```python
from build123d import *

# Parameters (mm, degrees)
SKETCH_1_W             = 68.22
SKETCH_1_H             = 22
SM_BASE_FLANGE_1_DEPTH = 1
FILLET_1_R             = 1
OTHER_START            = -15.667913645
OTHER_1_DEPTH          = 22
OTHER_1_2_DEPTH        = 22
OTHER_START_2          = 27.250753262
OTHER_1_3_DEPTH        = 1.749246738
SKETCH_7_R             = 2
CUT_EXTRUDE_1_DEPTH    = 40
SKETCH_7_6_R           = 1.7
CUT_EXTRUDE_4_DEPTH    = 20


with BuildPart() as part:
    # 基体-法兰1: sheet metal written as solids
    # Sketch 1 → 基体-法兰1 (new body)
    with BuildSketch(Plane(origin=(0, 0, 0), x_dir=(1, 0, 0), z_dir=(0, 1, 0))):
        with Locations((-53.201792275, 4.667913645)):
            Rectangle(SKETCH_1_W, SKETCH_1_H)
    extrude(amount=-SM_BASE_FLANGE_1_DEPTH)

    # 圆角1
    fillet_1_edges = [part.edges().sort_by_distance(p)[0] for p in [
        (-87.311792275, -0.5, -15.667913645),
        (-19.091792275, -0.5, -15.667913645),
        (-19.091792275, -0.5, 6.332086355),
        (-87.311792275, -0.5, 6.332086355),
    ]]
    fillet(fillet_1_edges, radius=FILLET_1_R)

    # Other 1: read off the stored shape, not the designer's step
    # Other 1 outline → Other 1 (cut)
    with BuildSketch(Plane.XY.offset(OTHER_START)):
        with BuildLine():
            Line((-19.091792275, 0), (-53.739151185, 0))
            ThreePointArc((-53.739151185, 0), (-54.379966111, -0.728828115), (-55.311792275, -1))
            Line((-55.311792275, -1), (-19.091792275, -1))
            Line((-19.091792275, -1), (-19.091792275, 0))
        make_face()
    extrude(amount=OTHER_1_DEPTH, mode=Mode.SUBTRACT)

    # Other 1 2 outline → Other 1 2 (add)
    with BuildSketch(Plane.XY.offset(OTHER_START)):
        with BuildLine():
            ThreePointArc((-53.739151185, 0), (-53.616677518, 0.359286442), (-53.575192275, 0.7366))
            Line((-53.575192275, 0.7366), (-53.575192275, 26.514153262))
            ThreePointArc((-53.575192275, 26.514153262), (-54.083830639, 27.742114898), (-55.311792275, 28.250753262))
            Line((-55.311792275, 28.250753262), (-61.869345538, 28.250753262))
            Line((-61.869345538, 28.250753262), (-61.869345538, 27.250753262))
            Line((-61.869345538, 27.250753262), (-55.311792275, 27.250753262))
            ThreePointArc((-55.311792275, 27.250753262), (-54.79093742, 27.035008117), (-54.575192275, 26.514153262))
            Line((-54.575192275, 26.514153262), (-54.575192275, 0.7366))
            ThreePointArc((-54.575192275, 0.7366), (-54.79093742, 0.215745145), (-55.311792275, 0))
            Line((-55.311792275, 0), (-53.739151185, 0))
        make_face()
    extrude(amount=OTHER_1_2_DEPTH)

    # Other 1 3 outline → Other 1 3 (cut)
    with BuildSketch(Plane(origin=(0, 0, 0), x_dir=(1, 0, 0), z_dir=(0, 1, 0)).offset(OTHER_START_2)):
        with BuildLine():
            Line((-61.869345538, -6.332086355), (-60.869345538, -6.332086355))
            ThreePointArc((-60.869345538, -6.332086355), (-61.576452319, -6.039193136), (-61.869345538, -5.332086355))
            Line((-61.869345538, -5.332086355), (-61.869345538, -6.332086355))
        make_face()
        with BuildLine():
            Line((-61.869345538, 15.667913645), (-61.869345538, 14.667913645))
            ThreePointArc((-61.869345538, 14.667913645), (-61.576452319, 15.375020426), (-60.869345538, 15.667913645))
            Line((-60.869345538, 15.667913645), (-61.869345538, 15.667913645))
        make_face()
    extrude(amount=OTHER_1_3_DEPTH, mode=Mode.SUBTRACT)

    # 草图7 → 切除-拉伸1 (cut)
    with BuildSketch(Plane(origin=(0, 28.250753262, 0), x_dir=(1, 0, 0), z_dir=(0, 1, 0))):
        with Locations(Location((-80.654608631, -2.961737693, 0), (0, 0, 90))):
            Circle(SKETCH_7_R)
    extrude(amount=-CUT_EXTRUDE_1_DEPTH, mode=Mode.SUBTRACT)

    # 草图7<6> → 切除-拉伸4 (cut)
    with BuildSketch(Plane(origin=(0, 28.250753262, 0), x_dir=(1, 0, 0), z_dir=(0, 1, 0))):
        with Locations(Location((-58.548227621, 10.901663137, 0), (0, 0, 180))):
            Circle(SKETCH_7_6_R)
        with Locations(Location((-58.548227621, 0.801663137, 0), (0, 0, 180))):
            Circle(SKETCH_7_6_R)
    extrude(amount=-CUT_EXTRUDE_4_DEPTH, mode=Mode.SUBTRACT)


solid = part.part
```
Geometry check sheet. Reference: the model listing, model coordinates, mm. A direction names the side the tool comes from. Coordinates: 2 decimals unless noted, no trailing zeros. Order: outer loops, then holes, each group sorted by start corner. A loop starts at its lowest first (then second) coordinate and runs counter-clockwise, first axis right, second up.
Item 1: Tool access check on faces 1 (the cylindrical face through (-61.58, 27.74, -15.37)), 2 (the cylindrical face through (-61.569, 27.744, 6.047)), 3 (the cylindrical face through (-57.3, 27.76, -9.75)), 4 (the flat face through (-61.869, 28, -5)), 5 (the flat face through (-54.575, 14, -5)). Record the directions out of +Z, -Z, +X, -X, +Y, -Y that give a thin tool (end or side, any length) a straight path to the whole face; none if there is none.
Item 2: Depth check by flat-ended pin: pin 1 (6.5 mm diameter, centred on y = 13.5, z = -8.5, fed in from -X); pin 2 (3.5 mm diameter, centred on x = -80.65, z = 2.96, fed in from -Y); pin 3 (1.1 mm diameter, centred on y = 27.5, z = -7, fed in from -X). Enter the tip coordinate at first touch or a pass-through.
Item 3: Section check A-A (z = -13.75). Enter the section's corners in (x, y).
Item 4: Section check B-B (x = -71.5). Enter the section's corners in (y, z), plus the area to 3 significant figures.
Item 5: Section check C-C (y = 21.5). Enter the section's corners in (x, z), plus the area to 3 significant figures.
Item 6: Mould release check, pull along Y, two halves, no side actions. Record for faces 6 (the flat face through (-59, 27.251, -5)), 7 (the flat face through (-72, -1, -5)), 8 (the flat face through (-72, 0, -5)), 9 (the flat face through (-53.575, 13, -5)): released by +Y, released by -Y, zero draft, split by the parting line, or undercut.
Item 7: Scan lines: line 1 along Y through (x, z) = (-58, -8.5); line 2 along X through (y, z) = (16.5, -13); line 3 along Y through (x, z) = (-66, -9). Record each from-to range of solid material in increasing order.
Check sheet entries:
1. face 1: -Z, -X, +Y
1. face 2: +Z, -X, +Y
1. face 3: +Y
1. face 4: +Z, -Z, -X, +Y
1. face 5: +Z, -Z, -X
2. pin 1: stops at x = -54.58
2. pin 2: passes through
2. pin 3: stops at x = -61.87
3. outline: (-87.31, -1) - (-55.31, -1) arc R1.74 ccw to (-53.58, 0.74) - (-53.58, 26.51) arc R1.74 ccw to (-55.31, 28.25) - (-61.87, 28.25) - (-61.87, 27.25) - (-55.31, 27.25) arc R0.74 cw to (-54.58, 26.51) - (-54.58, 0.74) arc R0.74 cw to (-55.31, 0) - (-87.31, 0) - close
4. outline: (-1, -15.67) - (0, -15.67) - (0, 6.33) - (-1, 6.33) - close
4. area: 22.0 mm2
5. outline: (-54.58, -15.67) - (-53.58, -15.67) - (-53.58, 6.33) - (-54.58, 6.33) - close
5. area: 22.0 mm2
6. face 6: undercut
6. face 7: released by -Y
6. face 8: undercut
6. face 9: zero draft
7. line 1: y = -1 to 0, 27.25 to 28.25
7. line 2: x = -54.58 to -53.58
7. line 3: y = -1 to 0
